from build123d import *

# Parameters (mm, degrees)
PAD_DEPTH       = 6.85
PAD001_DEPTH    = 3.15
FILLET_R        = 1
FILLET001_R     = 1.5
SKETCH002_W     = 2
SKETCH002_H     = 8
PAD002_DEPTH    = 1
SKETCH003_W     = 2
SKETCH003_H     = 8
PAD003_DEPTH    = 1
SKETCH004_R     = 2.5
POCKET_DEPTH    = 4.151
SKETCH005_R     = 2.5
POCKET001_DEPTH = 4.151


with BuildPart() as part:
    # Sketch → Pad (new body, symmetric)
    with BuildSketch(Plane.YZ):
        Polygon((0, 28), (0, 5), (5, 5), (5, 0), (28, 0), (28, 3.15), (8.15, 3.15), (8.15, 8.15), (3.15, 8.15), (3.15, 28), align=None)
    extrude(amount=PAD_DEPTH, both=True)

    # Sketch001 (on Face11 of Pad) → Pad001 (join)
    with BuildSketch(Plane(origin=(-6.85, 0, 0), x_dir=(0, 1, 0), z_dir=(-1, 0, 0))):
        Polygon((0, -28), (0, -5), (5, -5), (5, 0), (28, 0), (28, -3.15), (3.15, -28), align=None)
    pad001 = extrude(amount=PAD001_DEPTH)

    # Mirrored: Pad001 across YZ
    add(pad001.mirror(Plane.YZ))

    # Fillet
    fillet_edges = [part.edges().sort_by_distance(p)[0] for p in [
        (0, 5, 0),
        (0, 0, 5),
    ]]
    fillet(fillet_edges, radius=FILLET_R)

    # Fillet001
    fillet001_edges = [part.edges().sort_by_distance(p)[0] for p in [
        (0, 3.15, 8.15),
        (0, 8.15, 8.15),
        (0, 8.15, 3.15),
    ]]
    fillet(fillet001_edges, radius=FILLET001_R)

    # Sketch002 (on Face26 of Fillet001) → Pad002 (join)
    with BuildSketch(Plane(origin=(0, 0, 0), x_dir=(0, 0, -1), z_dir=(0, -1, 0))):
        with Locations((-26, 0)):
            Rectangle(SKETCH002_W, SKETCH002_H)
        with Locations((-7.1, 0)):
            Rectangle(SKETCH002_W, SKETCH002_H)
    extrude(amount=PAD002_DEPTH)

    # Sketch003 (on Face16 of Pad002) → Pad003 (join)
    with BuildSketch(Plane.YX):
        with Locations((7.1, 0)):
            Rectangle(SKETCH003_W, SKETCH003_H)
        with Locations((26, 0)):
            Rectangle(SKETCH003_W, SKETCH003_H)
    extrude(amount=PAD003_DEPTH)

    # Sketch004 (on Face6 of Pad003) → Pocket (cut, through all)
    with BuildSketch(Plane.ZX.offset(3.15)):
        with Locations((17, 0)):
            Circle(SKETCH004_R)
    extrude(amount=-POCKET_DEPTH, mode=Mode.SUBTRACT)

    # Sketch005 (on Face2 of Pocket) → Pocket001 (cut, through all)
    with BuildSketch(Plane(origin=(0, 0, 3.15), x_dir=(0, -1, 0), z_dir=(0, 0, 1))):
        with Locations((-17, 0)):
            Circle(SKETCH005_R)
    extrude(amount=-POCKET001_DEPTH, mode=Mode.SUBTRACT)


solid = part.part
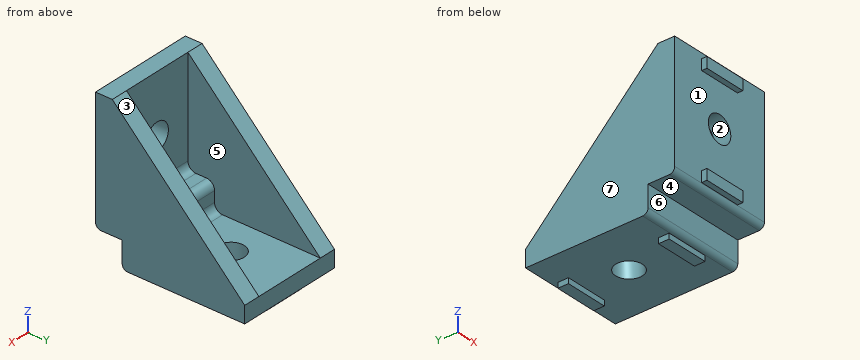
Can you work these out from the model? Positions are in its coordinate system, mm. Face numbers are marked on the shaded views. A direction names the side the tool comes from. Coordinates: 2 decimals unless noted, no trailing zeros. Loops run counter-clockwise (first coordinate to the right, second up) from the corner with the lowest first, then second, coordinate; pieces in that order, holes last. Notation, with made-up numbers: (75, 46.25) - (132, 46.25) arc R12 cw to (132, 66.25) - close; hole circle Ø2 at (77, 66). An arc over 180 degrees is marked (long way). Put each result on its own line as item: value. Start each with the question number.
Item 1: Suppose I cut it at C-C (y = 23). Please give me the cut outline in (x, z).
Item 2: Suppose I cut it at A-A (y = 17). Please give me the cut outline in (x, z), and give its area (3 significant figures).
Item 3: Suppose I cut it at D-D (x = -5.5). Please give me the cut outline in (y, z).
Item 4: If we mould it in two halves opening along Z, with no side actions, what happens to the marked faces 1, 2, 3 and 4? For each: +Z half, -Z half, draft (parallel to the pull), parting line (faces both ways), or undercut.
Item 5: For pin 1 (0.5 mm diameter, centred on x = 0, z = -0.5, fed in from -Y); pin 2 (0.5 mm diameter, centred on y = 26.5, z = -0.5, fed in from +X); pin 3 (3 mm diameter, centred on x = 2.5, z = 18, fed in from -Y), each with a flat end and sliding along its axis, tell me the tip position at first contact or that it passes through.
Item 6: Which directions (+Z, -Z, +X, -X, +Y, -Y) give clear straight access to the entire face, cutting with the end or side of a thin tool? Please do the marked faces 5, 6 and 7.
Item 7: If I drill on line 1 along X through (y, z) = (1.35, 17); line 2 along Y through (x, z) = (-4.5, 26.75); line 3 along X through (y, z) = (23.5, 6.25), over which ranges is the centre line in solid material (lowest first)?
Here are the results:
1. outline: (-10, 0) - (10, 0) - (10, 8.15) - (6.85, 8.15) - (6.85, 3.15) - (-6.85, 3.15) - (-6.85, 8.15) - (-10, 8.15) - close
2. outline: (-10, 0) - (-2.5, 0) - (-2.5, 3.15) - (-6.85, 3.15) - (-6.85, 14.15) - (-10, 14.15) - close; (2.5, 0) - (10, 0) - (10, 14.15) - (6.85, 14.15) - (6.85, 3.15) - (2.5, 3.15) - close
2. area: 117 mm²
3. outline: (0, 6) arc R1 ccw to (1, 5) - (5, 5) - (5, 1) arc R1 ccw to (6, 0) - (28, 0) - (28, 3.15) - (9.65, 3.15) arc R1.5 cw to (8.15, 4.65) - (8.15, 6.65) arc R1.5 ccw to (6.65, 8.15) - (4.65, 8.15) arc R1.5 cw to (3.15, 9.65) - (3.15, 28) - (0, 28) - close
4. face 1: undercut
4. face 2: undercut
4. face 3: +Z half
4. face 4: -Z half
5. pin 1: y = 6.1
5. pin 2: x = 4
5. pin 3: y = 0
6. face 5: +Z, +Y
6. face 6: -Z, +X, -X, -Y
6. face 7: +Z, -Z, -X, +Y, -Y
7. line 1: -10 to -2.5, 2.5 to 10
7. line 2: 0 to 3.15
7. line 3: -10 to -6.85, 6.85 to 10
